Geometry check sheet. Reference: the model listing, model coordinates, mm. A direction names the side the tool comes from. Coordinates: 2 decimals unless noted, no trailing zeros. Loops run counter-clockwise (first coordinate to the right, second up) from the corner with the lowest first, then second, coordinate; pieces in that order, holes last. Notation, with made-up numbers: M -24.5,26 L -8.5,26 A29 cw -8.5,55 Z; hole C -29.5,-11 d1. An arc over 180 degrees is marked long. Use CSV: the item, a comma, the result in double quotes.
```python
from build123d import *

# Parameters (mm, degrees)
SKETCH1_W           = 265
SKETCH1_H           = 62
BOSS_EXTRUDE1_DEPTH = 303
SHELL1_T            = -2
SKETCH2_W           = 265
SKETCH2_H           = 301
CUT_EXTRUDE1_DEPTH  = 50
SKETCH3_W           = 265
SKETCH3_H           = 2
BOSS_EXTRUDE2_DEPTH = 15


with BuildPart() as part:
    # Sketch1 → Boss-Extrude1 (new body)
    with BuildSketch(Plane.XY):
        Rectangle(SKETCH1_W, SKETCH1_H)
    extrude(amount=BOSS_EXTRUDE1_DEPTH)

    # Shell1
    shell1_openings = [part.faces().sort_by_distance(p)[0] for p in [
        (0, 31, 151.5),
    ]]
    offset(amount=SHELL1_T, openings=shell1_openings, kind=Kind.INTERSECTION)

    # Sketch2 → Cut-Extrude1 (cut)
    with BuildSketch(Plane(origin=(0, 31, 0), x_dir=(1, 0, 0), z_dir=(0, 1, 0))):
        with Locations((0, -150.5)):
            Rectangle(SKETCH2_W, SKETCH2_H)
    extrude(amount=-CUT_EXTRUDE1_DEPTH, mode=Mode.SUBTRACT)

    # Sketch3 → Boss-Extrude2 (add)
    with BuildSketch(Plane(origin=(0, 31, 0), x_dir=(1, 0, 0), z_dir=(0, 1, 0))):
        with Locations((0, -302)):
            Rectangle(SKETCH3_W, SKETCH3_H)
    extrude(amount=BOSS_EXTRUDE2_DEPTH)


solid = part.part
```
1. Section check C-C, the plane y = -0.5. Record the cut outline in (x, z), plus the area to 3 significant figures.
The answers:
outline,"M -132.5,301 L 132.5,301 L 132.5,303 L -132.5,303 Z"
area,"530 mm^2"
2. Section check A-A, the plane z = 122.5. Record the cut outline in (x, y).
The answers:
outline,"M -132.5,-31 L 132.5,-31 L 132.5,-19 L 130.5,-19 L 130.5,-29 L -130.5,-29 L -130.5,-19 L -132.5,-19 Z"
3. Section check B-B, the plane x = -91. Record the cut outline in (y, z), plus the area to 3 significant figures.
The answers:
outline,"M -31,0 L -19,0 L -19,2 L -29,2 L -29,301 L 46,301 L 46,303 L -31,303 Z"
area,"776 mm^2"
4. Release check for a two-part mould opening along Z. For faces 1 (the flat face through (-2, -24, 2)), 2 (the flat face through (-2, 7, 303)), 3 (the flat face through (-132.5, -27, 152)) record: +Z half, -Z half, draft (parallel to the pull), parting line (faces both ways), or undercut.
The answers:
face 1,"undercut"
face 2,"+Z half"
face 3,"draft"
5. Set-up check for faces 4 (the flat face through (132.5, -27, 152)), 5 (the flat face through (-130.5, -24, 149)): record each of +Z, -Z, +X, -X, +Y, -Y from which the full face is reachable in a straight line by a thin tool's end or side.
The answers:
face 4,"+Z, -Z, +X, +Y, -Y"
face 5,"+Y"
6. Thickness scan on line 1 (X direction, y = -25, z = 133.5); line 2 (Z direction, x = 8.5, y = -26); line 3 (Y direction, x = -25.5, z = 178.5). Record the ranges inside material, lowest first. Write a range as [from, to].
The answers:
line 1,"[-132.5, -130.5], [130.5, 132.5]"
line 2,"[0, 2], [301, 303]"
line 3,"[-31, -29]"
7. Gauge pin test, flat end, axial feed: P1, Ø4, axis at x = -92.5, y = 29.5, coming from the -Z side. Record the tip position at first contact, or that the pin passes through.
The answers:
P1,"z = 301"
